from build123d import *

# Parameters (mm, degrees)
SKETCH1_R               = 14.7
BOSS_EXTRUDE1_DEPTH     = 50
CUT_EXTRUDE1_REACH      = 56.15
SKETCH2_R               = 12.7
CUT_EXTRUDE2_REACH      = 60.88
CUT_EXTRUDE2_END_RADIUS = 12.7
SKETCH4_W               = 3.4
SKETCH4_H               = 50
SKETCH5_W               = 3.4
SKETCH5_H               = 6.4
CUT_EXTRUDE3_DEPTH      = 2
BOSS_EXTRUDE2_REACH     = 56.636
SKETCH7_W               = 3.4
SKETCH7_H               = 50
CUT_EXTRUDE4_DEPTH      = 0.114294
SKETCH8_W               = 3.4
SKETCH8_H               = 6.4
CUT_EXTRUDE5_DEPTH      = 2
BOSS_EXTRUDE3_REACH     = 56.636
SKETCH10_R              = 14.7
BOSS_EXTRUDE4_DEPTH     = 3.4
FILLET1_R               = 0.5
FILLET2_R               = 1


with BuildPart() as part:
    # Sketch1 → Boss-Extrude1 (new body)
    with BuildSketch(Plane(origin=(0, 0, 0), x_dir=(0, 1, 0), z_dir=(0, 0, 1))):
        with Locations(Location((0, 0, 0), (0, 0, 270))):
            Circle(SKETCH1_R)
    extrude(amount=BOSS_EXTRUDE1_DEPTH)

    # Sketch2 → Cut-Extrude1 (cut, up to next)
    with BuildSketch(Plane.XY.offset(50), mode=Mode.PRIVATE) as cut_extrude1_sk1:
        Circle(SKETCH2_R)
    cut_extrude1_tool1 = extrude(cut_extrude1_sk1.sketch, amount=-CUT_EXTRUDE1_REACH, mode=Mode.PRIVATE) & part.part
    add(cut_extrude1_tool1.solids().sort_by_distance((0, 0, 50))[0], mode=Mode.SUBTRACT)

    # Cut-Extrude2: up to this cylinder (the profile starts outside it)
    cut_extrude2_end = Plane(origin=(0, 0, 25), z_dir=(0, 0, 1)) * Cylinder(CUT_EXTRUDE2_END_RADIUS, 148.16, mode=Mode.PRIVATE)
    # Sketch4 → Cut-Extrude2 (cut, up to the surface)
    with BuildSketch(Plane(origin=(0, -12.7, 0), x_dir=(-1, 0, 0), z_dir=(0, 1, 0)), mode=Mode.PRIVATE) as cut_extrude2_sk1:
        with Locations((0, 25)):
            Rectangle(SKETCH4_W, SKETCH4_H)
    cut_extrude2_tool1 = extrude(cut_extrude2_sk1.sketch, amount=CUT_EXTRUDE2_REACH, mode=Mode.PRIVATE) - cut_extrude2_end
    add(cut_extrude2_tool1.solids().sort_by_distance((0, -12.7, 25))[0], mode=Mode.SUBTRACT)
    add(cut_extrude2_tool1.solids().sort_by_distance((0, -12.7, 25))[1], mode=Mode.SUBTRACT)

    # Sketch5 → Cut-Extrude3 (cut)
    with BuildSketch(Plane(origin=(0, -12.7, 0), x_dir=(-1, 0, 0), z_dir=(0, 1, 0))):
        with Locations((0, 30.973847717)):
            Rectangle(SKETCH5_W, SKETCH5_H)
    extrude(amount=-CUT_EXTRUDE3_DEPTH, mode=Mode.SUBTRACT)

    # Sketch6 → Boss-Extrude2 (add, up to next)
    with BuildSketch(Plane.YZ.offset(-1.7), mode=Mode.PRIVATE) as boss_extrude2_sk1:
        Polygon((-14.601369799, 27.773847717), (-12.7, 27.773847717), (-14.601369799, 29.675217516), align=None)
    boss_extrude2_tool1 = extrude(boss_extrude2_sk1.sketch, amount=BOSS_EXTRUDE2_REACH, mode=Mode.PRIVATE) - part.part
    # Sketch6 → Boss-Extrude2 (add, up to next)
    with BuildSketch(Plane.YZ.offset(-1.7), mode=Mode.PRIVATE) as boss_extrude2_sk2:
        Polygon((-14.601369799, 34.173847717), (-12.7, 34.173847717), (-14.601369799, 32.272477918), align=None)
    boss_extrude2_tool2 = extrude(boss_extrude2_sk2.sketch, amount=BOSS_EXTRUDE2_REACH, mode=Mode.PRIVATE) - part.part
    add(boss_extrude2_tool1.solids().sort_by_distance((-1.7, -13.96758, 28.407638))[0])
    add(boss_extrude2_tool2.solids().sort_by_distance((-1.7, -13.96758, 33.540058))[0])

    # Sketch7 → Cut-Extrude4 (cut)
    with BuildSketch(Plane.XZ.offset(-12.7)):
        with Locations((0, 25)):
            Rectangle(SKETCH7_W, SKETCH7_H)
    extrude(amount=CUT_EXTRUDE4_DEPTH, mode=Mode.SUBTRACT)

    # Sketch8 → Cut-Extrude5 (cut)
    with BuildSketch(Plane.XZ.offset(-12.7)):
        with Locations((0, 30.973847717)):
            Rectangle(SKETCH8_W, SKETCH8_H)
    extrude(amount=-CUT_EXTRUDE5_DEPTH, mode=Mode.SUBTRACT)

    # Sketch9 → Boss-Extrude3 (add, up to next)
    with BuildSketch(Plane.YZ.offset(-1.7), mode=Mode.PRIVATE) as boss_extrude3_sk1:
        Polygon((14.601369799, 34.173847717), (14.601369799, 32.272477918), (12.7, 34.173847717), align=None)
    boss_extrude3_tool1 = extrude(boss_extrude3_sk1.sketch, amount=BOSS_EXTRUDE3_REACH, mode=Mode.PRIVATE) - part.part
    # Sketch9 → Boss-Extrude3 (add, up to next)
    with BuildSketch(Plane.YZ.offset(-1.7), mode=Mode.PRIVATE) as boss_extrude3_sk2:
        Polygon((14.601369799, 27.773847717), (14.601369799, 29.675217516), (12.7, 27.773847717), align=None)
    boss_extrude3_tool2 = extrude(boss_extrude3_sk2.sketch, amount=BOSS_EXTRUDE3_REACH, mode=Mode.PRIVATE) - part.part
    add(boss_extrude3_tool1.solids().sort_by_distance((-1.7, 13.96758, 33.540058))[0])
    add(boss_extrude3_tool2.solids().sort_by_distance((-1.7, 13.96758, 28.407638))[0])

    # Sketch10 → Boss-Extrude4 (add)
    with BuildSketch(Plane.XY.offset(50)):
        Circle(SKETCH10_R)
    extrude(amount=BOSS_EXTRUDE4_DEPTH)

    # Fillet1
    fillet1_edges = [part.edges().sort_by_distance(p)[0] for p in [
        (0, 12.7, 27.773847717),
        (0, 12.7, 34.173847717),
        (0, 14.601369799, 32.272477918),
        (0, 14.601369799, 29.675217516),
        (0, -12.7, 27.773847717),
        (0, -12.7, 34.173847717),
        (0, -14.601369799, 29.675217516),
        (0, -14.601369799, 32.272477918),
    ]]
    fillet(fillet1_edges, radius=FILLET1_R)

    # Fillet2
    fillet2_edges = [part.edges().sort_by_distance(p)[0] for p in [
        (-14.7, 0, 53.4),
    ]]
    fillet(fillet2_edges, radius=FILLET2_R)


solid = part.part
Input: part model. Units: mm. Frame: model coordinates. A direction names the side the tool comes from. Coordinates: 2 decimals unless noted, no trailing zeros. Loops run counter-clockwise (first coordinate to the right, second up) from the corner with the lowest first, then second, coordinate; pieces in that order, holes last. Notation, with made-up numbers: (6, 31) -> (45, 31) arc R29 cw to (45, 55) -> close; hole circle Ø7 at (47.25, 22.5). An arc over 180 degrees is marked (long way). Write item = value, one per line. Start each with the question number.
Item 1: First-contact query: P1, Ø12.5, axis at x = -0.5, y = 6, coming from the -Z side; P2, Ø0.6, axis at x = -0.5, z = 28, coming from the +Y side; P3, Ø8, axis at y = -4.5, z = 7, coming from the -X side. Flat tips, straight axial feed; report the tip coordinate or a pass-through.
Item 2: Mould query, pull axis X, two halves, no side actions, for faces 1 (the face through (-13, 0, 0)), 2 (the face through (0, -12.7, 14)), 3 (the face through (-3.19, -14.35, 25.83)). Classes: pulls with the +X half, pulls with the -X half, needs draft (parallel to the pull), parting line crosses it, or undercut.
Item 3: Reachability of faces 4 (the face through (0, 0, 53.4)), 5 (the face through (1.7, -13, 29)), 6 (the face through (12.697, -0.255, 25.35)) from +Z, -Z, +X, -X, +Y, -Y: full face, straight path, thin tool, end or side. Return the list, or none.
Item 4: Cut plane B-B, the plane z = 43.5. Return loops of the section in (x, y), plus the area to 3 significant figures.
Item 5: Cut plane A-A, the plane x = 0. Count the separate pieces of the cut face and the enclosed holes in it, plus the area to 3 significant figures.
Item 6: Cut plane C-C, the plane y = 0. Return loops of the section in (x, z).
Item 7: Material intervals for line 1 (X direction, y = -0.25, z = 23); line 2 (Y direction, x = -0.5, z = 9.5); line 3 (Z direction, x = -0.5, y = -3.5), sorted ascending.
Ans:
q1.P1 = 50
q1.P2 = 14.7
q1.P3 = -14.69
q2.face_1 = needs draft
q2.face_2 = undercut
q2.face_3 = parting line crosses it
q3.face_4 = +Z, +X, -X, +Y, -Y
q3.face_5 = none
q3.face_6 = -Z
q4.outline = circle Ø29.4 at (0, 0); hole (-1.7, -12.7) -> (1.7, -12.7) -> (1.7, -12.59) arc R12.7 ccw to (1.7, 12.59) -> (1.7, 12.7) -> (-1.7, 12.7) -> (-1.7, 12.59) arc R12.7 ccw to (-1.7, -12.59) -> close
q4.area = 172 mm²
q5.separate_pieces = 3
q5.enclosed_holes = 0
q5.area = 280 mm²
q6.outline = (-14.7, 0) -> (-12.7, 0) -> (-12.7, 50) -> (12.7, 50) -> (12.7, 0) -> (14.7, 0) -> (14.7, 52.4) arc R1 ccw to (13.7, 53.4) -> (-13.7, 53.4) arc R1 ccw to (-14.7, 52.4) -> close
q7.line_1 = -14.7 to -12.7, 12.7 to 14.7
q7.line_2 = -14.69 to -12.7, 12.7 to 14.69
q7.line_3 = 50 to 53.4
